Input: part model. Units: mm. Frame: model coordinates. A direction names the side the tool comes from. Coordinates: 2 decimals unless noted, no trailing zeros. Loops run counter-clockwise (first coordinate to the right, second up) from the corner with the lowest first, then second, coordinate; pieces in that order, holes last. Notation, with made-up numbers: (-2, 29) -> (49, 29) arc R21 cw to (49, 56) -> close; hole circle Ø5 at (80, 73). An arc over 180 degrees is marked (long way). Put each result on its own line as item: value. Start each with the question number.
1) Cut plane B-B (y = -7.5). Return the cut outline in (x, z) (1 decimal).
2) Cut plane C-C (x = -20). Return the cut outline in (y, z), plus the area to 3 significant figures.
3) Contact query for flat-ended pins moving along their axis: P1, Ø5, axis at x = -14, z = -7, coming from the +Y side; P2, Ø2, axis at y = -9.5, z = -7.5, coming from the +X side; P3, Ø2, axis at x = 13.5, z = -5, coming from the -Y side. Output: stop coordinate, or through.
4) Cut plane D-D (y = -22). Return the cut outline in (x, z) (1 decimal).
5) Pull-direction query (Z, two-part tool) for faces 3 (the flat face through (-30.117, -11, -6)), 4 (the flat face through (-26, -9, -2.381)), 5 (the flat face through (0, 4, -11.112)); classes: pulls with the +Z half, pulls with the -Z half, needs draft (parallel to the pull), parting line crosses it, or undercut.
6) Material intervals for L1, parallel to Z at x = -12, y = 4; L2, parallel to X at y = -9.5, z = -2.25; L3, parallel to Z at x = -27.5, y = -10.5 (1 decimal), sorted ascending.
7) Cut plane A-A (z = -5.25). Return the cut outline in (x, y).
8) Set-up query: faces 1 (the flat face through (28, -14, -9.525)), 2 (the flat face through (29, -24.954, -10)). Return all of +Z, -Z, +X, -X, +Y, -Y with unobstructed straight access to the full face (end or side cutting, diameter ignored); none if empty.
from build123d import *

# Parameters (mm, degrees)
BOSS_EXTRUDE1_DEPTH              = 12.7
SKETCH3_W                        = 4.569606656
SKETCH3_H                        = 12.610946307
CUT_EXTRUDE1_DEPTH               = 32.573497659
CUT_EXTRUDE1_DEPTH_BACK          = 32.704428158
SKETCH4_W                        = 4.569606656
SKETCH4_H                        = 7.9375
CUT_EXTRUDE2_DEPTH               = 66.04
SKETCH5_W                        = 1.5875
SKETCH5_H                        = 39.725965327
CUT_EXTRUDE3_DEPTH               = 32.573497659
CUT_EXTRUDE3_DEPTH_BACK          = 32.704428158
SKETCH6_W                        = 1.5875
SKETCH6_H                        = 40.415060451
CUT_EXTRUDE4_DEPTH               = 0.79375
SKETCH7_W                        = 1.5875
SKETCH7_H                        = 38.718479636
SKETCH7_H_2                      = 39.708151778
CUT_EXTRUDE5_DEPTH               = 0.79375
CUT_EXTRUDE6_REACH               = 9.892
CUT_EXTRUDE6_OFFSET_FROM_SURFACE = 1.5875
SKETCH8_W                        = 6.35
SKETCH8_H                        = 22.490762182
SKETCH9_W                        = 6.35
SKETCH9_H                        = 22.482269966
CUT_EXTRUDE7_DEPTH               = 5.55625
SKETCH10_W                       = 0.79375
SKETCH10_H                       = 36.880517087
CUT_EXTRUDE8_DEPTH               = 12.1125


with BuildPart() as part:
    # Sketch1 → Boss-Extrude1 (new body)
    with BuildSketch(Plane.XY):
        with BuildLine():
            Line((25.223497659, -24.95432425), (31.573497659, -24.95432425))
            Line((31.573497659, -24.95432425), (31.573497659, 0.44567575))
            ThreePointArc((31.573497659, 0.44567575), (29.713625719, 4.935803811), (25.223497659, 6.79567575))
            Line((25.223497659, 6.79567575), (25.223497659, 3.36874218))
            ThreePointArc((25.223497659, 3.36874218), (25.194005143, 3.37526688), (25.164511033, 3.381784371))
            ThreePointArc((25.164511033, 3.381784371), (23.912297459, 5.232947026), (22.049913461, 3.997484421))
            ThreePointArc((22.049913461, 3.997484421), (20.787428344, 5.879791305), (18.929672437, 4.581449722))
            ThreePointArc((18.929672437, 4.581449722), (17.666399498, 6.401938478), (15.813867684, 5.186140916))
            ThreePointArc((15.813867684, 5.186140916), (14.370419451, 6.86745546), (12.652448322, 5.467835298))
            ThreePointArc((12.652448322, 5.467835298), (11.236710182, 7.228730664), (9.494148573, 5.790486593))
            ThreePointArc((9.494148573, 5.790486593), (8.033635968, 7.514426817), (6.328601682, 6.03188675))
            ThreePointArc((6.328601682, 6.03188675), (4.824278861, 7.717733664), (3.157897585, 6.191876393))
            ThreePointArc((3.157897585, 6.191876393), (1.610757722, 7.838516978), (-0.015870376, 6.270349895))
            ThreePointArc((-0.015870376, 6.270349895), (-1.604805836, 7.876697016), (-3.190606835, 6.267255447))
            ThreePointArc((-3.190606835, 6.267255447), (-4.820288856, 7.832248571), (-6.364215787, 6.182595092))
            ThreePointArc((-6.364215787, 6.182595092), (-8.033568431, 7.705200989), (-9.534601973, 6.016424724))
            ThreePointArc((-9.534601973, 6.016424724), (-11.24252311, 7.495638149), (-12.69967226, 5.76885405))
            ThreePointArc((-12.69967226, 5.76885405), (-14.466077033, 7.201365285), (-15.851850507, 5.398061056))
            ThreePointArc((-15.851850507, 5.398061056), (-17.628014087, 6.745603643), (-18.999984081, 4.988240156))
            ThreePointArc((-18.999984081, 4.988240156), (-20.801252814, 6.376658399), (-22.142035626, 4.539656571))
            ThreePointArc((-22.142035626, 4.539656571), (-23.987693231, 5.836740457), (-25.266933007, 3.978670437))
            ThreePointArc((-25.266933007, 3.978670437), (-25.282113604, 3.97569181), (-25.297293828, 3.972711283))
            Line((-25.297293828, 3.972711283), (-25.297293828, 6.794845101))
            ThreePointArc((-25.297293828, 6.794845101), (-29.574532825, 5.2306288), (-31.704428158, 1.205073937))
            Line((-31.704428158, 1.205073937), (-31.704428158, -24.95432425))
            Line((-31.704428158, -24.95432425), (-25.4, -24.95432425))
            Line((-25.4, -24.95432425), (-25.440666935, -2.463598833))
            ThreePointArc((-25.440666935, -2.463598833), (-0.075359426, 0.000928604), (25.223497659, -3.071619312))
            Line((25.223497659, -3.071619312), (25.223497659, -24.95432425))
        make_face()
    extrude(amount=-BOSS_EXTRUDE1_DEPTH)

    # Sketch3 → Cut-Extrude1 (cut, two sides)
    with BuildSketch(Plane(origin=(0, 0, 0), x_dir=(0, 0, -1), z_dir=(1, 0, 0))) as cut_extrude1_sk:
        with Locations((6.35, 6.751148903)):
            Rectangle(SKETCH3_W, SKETCH3_H)
    extrude(amount=CUT_EXTRUDE1_DEPTH, mode=Mode.SUBTRACT)
    extrude(cut_extrude1_sk.sketch, amount=-CUT_EXTRUDE1_DEPTH_BACK, mode=Mode.SUBTRACT)

    # Sketch4 → Cut-Extrude2 (cut)
    with BuildSketch(Plane(origin=(31.573497659, 0, 0), x_dir=(0, 0, -1), z_dir=(1, 0, 0))):
        with Locations((6.35, -19.39807425)):
            Rectangle(SKETCH4_W, SKETCH4_H)
    extrude(amount=-CUT_EXTRUDE2_DEPTH, mode=Mode.SUBTRACT)

    # Sketch5 → Cut-Extrude3 (cut, two sides)
    with BuildSketch(Plane(origin=(0, 0, 0), x_dir=(0, 0, -1), z_dir=(1, 0, 0))) as cut_extrude3_sk:
        with Locations((0.79375, -5.091341587)):
            Rectangle(SKETCH5_W, SKETCH5_H)
        with Locations((11.90625, -5.091341587)):
            Rectangle(SKETCH5_W, SKETCH5_H)
    extrude(amount=CUT_EXTRUDE3_DEPTH, mode=Mode.SUBTRACT)
    extrude(cut_extrude3_sk.sketch, amount=-CUT_EXTRUDE3_DEPTH_BACK, mode=Mode.SUBTRACT)

    # Sketch6 → Cut-Extrude4 (cut)
    with BuildSketch(Plane.XY.offset(-1.5875)):
        with Locations((26.017247659, -4.746794025)):
            Rectangle(SKETCH6_W, SKETCH6_H)
        with Locations((-26.017247659, -4.746794025)):
            Rectangle(SKETCH6_W, SKETCH6_H)
    extrude(amount=-CUT_EXTRUDE4_DEPTH, mode=Mode.SUBTRACT)

    # Sketch7 → Cut-Extrude5 (cut)
    with BuildSketch(Plane(origin=(0, 0, -11.1125), x_dir=(-1, 0, 0), z_dir=(0, 0, -1))):
        with Locations((26.19375, -5.595084432)):
            Rectangle(SKETCH7_W, SKETCH7_H)
        with Locations((-26.017247659, -5.100248361)):
            Rectangle(SKETCH7_W, SKETCH7_H_2)
    extrude(amount=-CUT_EXTRUDE5_DEPTH, mode=Mode.SUBTRACT)

    # Cut-Extrude6: up to this face of the body (flat: up to its plane, moved by the offset)
    cut_extrude6_end = Plane(part.part.faces().sort_by_distance((-31.704428158, -10.78205278, -6.35))[0]).offset(-CUT_EXTRUDE6_OFFSET_FROM_SURFACE)
    # Sketch8 → Cut-Extrude6 (cut, up to the picked face)
    with BuildSketch(Plane(origin=(-25.445038336, -0.046008819, 0), x_dir=(0, 0, -1), z_dir=(0.999998365, 0.001808162, 0)), mode=Mode.PRIVATE) as cut_extrude6_sk1:
        with Locations((6.35, -13.662975058)):
            Rectangle(SKETCH8_W, SKETCH8_H)
    cut_extrude6_tool1 = split(extrude(cut_extrude6_sk1.sketch, amount=-CUT_EXTRUDE6_REACH, mode=Mode.PRIVATE), bisect_by=cut_extrude6_end, keep=Keep.BOTH, mode=Mode.PRIVATE)
    add(cut_extrude6_tool1.solids().sort_by_distance((-25.420333, -13.708962, -6.35))[0], mode=Mode.SUBTRACT)

    # Sketch9 → Cut-Extrude7 (cut)
    with BuildSketch(Plane.ZY.offset(-25.223497659)):
        with Locations((-6.35, -13.713189267)):
            Rectangle(SKETCH9_W, SKETCH9_H)
    extrude(amount=-CUT_EXTRUDE7_DEPTH, mode=Mode.SUBTRACT)

    # Sketch10 → Cut-Extrude8 (cut, through all)
    with BuildSketch(Plane.XY):
        Polygon((-31.704428158, -24.691676413), (-31.704428158, 9.381321615), (-30.910678158, 9.381321615), (-30.910678158, -24.691676413), (-30.910678158, -24.95432425), (-31.704428158, -24.95432425), align=None)
        with Locations((31.176622659, -6.514065707)):
            Rectangle(SKETCH10_W, SKETCH10_H)
    extrude(amount=-CUT_EXTRUDE8_DEPTH, mode=Mode.SUBTRACT)


solid = part.part
Results found:
1. outline: (-30.9, -11.1) -> (-27, -11.1) -> (-27, -10.3) -> (-25.4, -10.3) -> (-25.4, -9.5) -> (-30.1, -9.5) -> (-30.1, -3.2) -> (-25.4, -3.2) -> (-25.4, -2.4) -> (-26.8, -2.4) -> (-26.8, -1.6) -> (-30.9, -1.6) -> close; (25.2, -10.3) -> (26.8, -10.3) -> (26.8, -11.1) -> (30.8, -11.1) -> (30.8, -9.5) -> (25.2, -9.5) -> close; (25.2, -3.2) -> (30.8, -3.2) -> (30.8, -1.6) -> (26.8, -1.6) -> (26.8, -2.4) -> (25.2, -2.4) -> close
2. outline: (-1.46, -11.11) -> (6.28, -11.11) -> (6.28, -8.63) -> (0.45, -8.63) -> (0.45, -4.07) -> (6.28, -4.07) -> (6.28, -1.59) -> (-1.46, -1.59) -> close
2. area: 47.1 mm2
3. P1: stops at y = 7.21
3. P2: stops at x = -30.12
3. P3: stops at y = -1.08
4. outline: (-30.9, -11.1) -> (-27, -11.1) -> (-27, -10.3) -> (-25.4, -10.3) -> (-25.4, -9.5) -> (-30.1, -9.5) -> (-30.1, -8.6) -> (-30.9, -8.6) -> close; (-30.9, -4.1) -> (-30.1, -4.1) -> (-30.1, -3.2) -> (-25.4, -3.2) -> (-25.4, -2.4) -> (-26.8, -2.4) -> (-26.8, -1.6) -> (-30.9, -1.6) -> close; (25.2, -10.3) -> (26.8, -10.3) -> (26.8, -11.1) -> (30.8, -11.1) -> (30.8, -9.5) -> (25.2, -9.5) -> close; (25.2, -3.2) -> (30.8, -3.2) -> (30.8, -1.6) -> (26.8, -1.6) -> (26.8, -2.4) -> (25.2, -2.4) -> close
5. face 3: undercut
5. face 4: pulls with the +Z half
5. face 5: pulls with the -Z half
6. L1: z = -11.11 to -8.63, -4.07 to -1.59
6. L2: x = -30.91 to -26.81, 26.81 to 30.78
6. L3: z = -11.1 to -9.5, -3.2 to -1.6
7. outline: (-30.91, -24.95) -> (-30.12, -24.95) -> (-30.12, -23.37) -> (-30.91, -23.37) -> close; (-30.91, -15.43) -> (-30.12, -15.43) -> (-30.12, -2.47) -> (-25.44, -2.46) arc R117.29 cw to (25.22, -3.07) -> (25.22, -2.47) -> (30.78, -2.47) -> (30.78, 0.45) -> (-30.91, 0.45) -> close
8. face 1: +X, -Y
8. face 2: +Z, -Z, +X, -X, -Y
